The listing builds one solid part. Answer for the finished solid, in the listing's coordinates (mm). A direction names the side the tool comes from. Give positions to 0.01 mm unless a question says otherwise; leave off trailing zeros. Loops run counter-clockwise (first coordinate to the right, second up) from the corner with the lowest first, then second, coordinate; pieces in that order, holes last. Notation, with made-up numbers: M 35.5,-10.5 L 40.5,-10.5 A26 cw 40.5,16.5 Z; hole C 19.5,15.5 d2. An arc over 180 degrees is marked long. One line per item, written item: value. Start each with the question number.
Q1. Consider L1, parallel to Z at x = -1, y = -10; L2, parallel to Z at x = 24, y = 6; L3, parallel to Y at x = 0, z = -9.8. Determine where each line is inside the solid, lowest interval first.
Q2. Flat-ended cylindrical pins translate along their axes: pin 1 (1.5 mm diameter, centred on y = -2, z = -5.5, fed in from -X); pin 2 (2.5 mm diameter, centred on x = 69.5, y = 0.5, fed in from +Z) (3 decimals); pin 3 (6.5 mm diameter, centred on x = 52, z = -4, fed in from +Y). Find the tip coordinate at first contact, or state that the pin passes through.
Q3. A cutting plane is placed at B-B, the plane y = 10.5. Determine the outline of the cut face in (x, z).
Q4. The mould has two halves that part along X. Classify faces 4 (the flat face through (6, 12.5, 2)), 5 (the flat face through (118, -3.2, -2.4)), 6 (the flat face through (48.56, -4.54, 1)): +X half, -X half, draft (parallel to the pull), parting line (faces both ways), or undercut.
Q5. For faces 1 (the flat face through (80, -1.5, 1)), 2 (the flat face through (81, 2, -0.35)), 3 (the flat face through (76, 0, -6.525)), determine the directions among +Z, -Z, +X, -X, +Y, -Y from which every point of the face is accessible in a straight line to the end or side of a thin tool.
Q6. A cutting plane is placed at A-A, the plane x = 96.5. Determine the outline of the cut face in (y, z) (3 decimals).
from build123d import *
from OCP.BRepFilletAPI import BRepFilletAPI_MakeChamfer
from build123d.topology import SkipClean

# Parameters (mm, degrees)
SKETCH1_R           = 7.0625
BOSS_EXTRUDE1_DEPTH = 4
SKETCH5_W           = 25.521905645
SKETCH5_H           = 15
BOSS_EXTRUDE2_DEPTH = 12.7
FILLET1_R           = 7.5
SKETCH6_W           = 64.371907972
SKETCH6_H           = 15
BOSS_EXTRUDE3_DEPTH = 2
CHAMFER1_SIZE       = 10
CHAMFER1_SIZE2      = 6
CHAMFER2_SIZE       = 6
CHAMFER2_SIZE2      = 10
SKETCH8_R           = 2.9375
BOSS_EXTRUDE4_DEPTH = 5
BOSS_EXTRUDE5_DEPTH = 1.5
CUT_EXTRUDE1_DEPTH  = 7.5
SKETCH11_W          = 6.742622272
SKETCH11_H          = 8.688704154
BOSS_EXTRUDE7_DEPTH = 8
FILLET2_R           = 2.5
SKETCH12_R          = 12.5
SKETCH12_R_2        = 7.0625
BOSS_EXTRUDE8_DEPTH = 1.5


# Some blends are built 0.0001 mm under size
with BuildPart() as part:
    # Sketch1 → Boss-Extrude1 (new body)
    with BuildSketch(Plane.XY):
        with BuildLine():
            Line((0, 12.5), (12.041321952, 12.5))
            Line((12.041321952, 12.5), (28.106186383, 7.5))
            Line((28.106186383, 7.5), (28.106186383, -7.5))
            Line((28.106186383, -7.5), (12.041321952, -12.5))
            Line((12.041321952, -12.5), (0, -12.5))
            ThreePointArc((0, -12.5), (-12.5, 0), (0, 12.5))
        make_face()
        Circle(SKETCH1_R, mode=Mode.SUBTRACT)
    boss_extrude1 = extrude(amount=BOSS_EXTRUDE1_DEPTH)

    # Sketch5 → Boss-Extrude2 (add)
    with BuildSketch(Plane.XY.offset(4)):
        with Locations((40.867139206, 0)):
            Rectangle(SKETCH5_W, SKETCH5_H)
    extrude(amount=-BOSS_EXTRUDE2_DEPTH)

    # Mirror1: Boss-Extrude1 across plane
    add(boss_extrude1.mirror(Plane(origin=(0, 0, -2.35), x_dir=(1, 0, 0), z_dir=(0, 0, -1))))

    # Fillet1
    fillet1_edges = [part.edges().sort_by_distance(p)[0] for p in [
        (28.106186383, -7.5, -2.35),
        (28.106186383, 7.5, -2.35),
    ]]
    fillet(fillet1_edges, radius=FILLET1_R - 0.0001)  # a hair under: the kernel refuses the full size

    # Sketch6 → Boss-Extrude3 (add, symmetric)
    with BuildSketch(Plane(origin=(0, 0, -2.35), x_dir=(-1, 0, 0), z_dir=(0, 0, -1))):
        with Locations((-85.814046014, 0)):
            Rectangle(SKETCH6_W, SKETCH6_H)
    extrude(amount=BOSS_EXTRUDE3_DEPTH, both=True)

    # Chamfer1
    chamfer1_edges = [part.edges().sort_by_distance(p)[0] for p in [
        (53.628092028, 7.5, -6.525),
        (53.628092028, 7.5, 1.825),
    ]]
    chamfer1_side = [part.faces().sort_by_distance(p)[0] for p in [
        (62.630754808, 7.5, -2.35),
    ]]
    chamfer(chamfer1_edges, length=CHAMFER1_SIZE, length2=CHAMFER1_SIZE2, reference=chamfer1_side[0])

    # Chamfer2: one chamfer whose edges measure the first distance from different faces: ONE call of the kernel's chamfer builder (chamfer() names one face for all edges)
    chamfer2_edges_1 = [part.edges().sort_by_distance(p)[0] for p in [
        (53.628092028, -7.5, -6.525),
    ]]
    chamfer2_side_1 = [part.faces().sort_by_distance(p)[0] for p in [
        (53.628092028, -3, -6.525),
    ]]
    chamfer2_edges_2 = [part.edges().sort_by_distance(p)[0] for p in [
        (53.628092028, -7.5, 1.825),
    ]]
    chamfer2_side_2 = [part.faces().sort_by_distance(p)[0] for p in [
        (53.628092028, -3, 1.825),
    ]]
    chamfer2 = BRepFilletAPI_MakeChamfer(part.part.solid().wrapped)
    for e in chamfer2_edges_1:
        chamfer2.Add(CHAMFER2_SIZE, CHAMFER2_SIZE2, e.wrapped, chamfer2_side_1[0].wrapped)  # the first distance lies on this face
    for e in chamfer2_edges_2:
        chamfer2.Add(CHAMFER2_SIZE, CHAMFER2_SIZE2, e.wrapped, chamfer2_side_2[0].wrapped)  # the first distance lies on this face
    add(Compound.cast(chamfer2.Shape()), mode=Mode.REPLACE)

    # Sketch8 → Boss-Extrude4 (add)
    with BuildSketch(Plane(origin=(118, 0, 0), x_dir=(0, 0, -1), z_dir=(1, 0, 0))):
        with Locations(Location((2.35, 0, 0), (0, 0, 132.910184022))):
            Circle(SKETCH8_R)
    extrude(amount=BOSS_EXTRUDE4_DEPTH)

    # Sketch9 → Boss-Extrude5 (add, symmetric)
    with BuildSketch(Plane(origin=(0, 0, 0), x_dir=(1, 0, 0), z_dir=(0, 1, 0))):
        Polygon((53.628092028, 6.525), (98.349917778, 6.525), (112.85605343, 2.35), (98.349917778, -1.825), (53.628092028, -1.825), align=None)
    extrude(amount=BOSS_EXTRUDE5_DEPTH, both=True)

    # Sketch10 → Cut-Extrude1 (cut, symmetric)
    with BuildSketch(Plane(origin=(0, 0, 0), x_dir=(1, 0, 0), z_dir=(0, 1, 0))):
        Polygon((53.628092028, 6.525), (35.842858925, 8.7), (53.628092028, 8.7), align=None)
        Polygon((53.628092028, -1.825), (35.842858925, -4), (53.628092028, -4), align=None)
    extrude(amount=CUT_EXTRUDE1_DEPTH, both=True, mode=Mode.SUBTRACT)

    # Sketch11 → Boss-Extrude7 (add)
    with BuildSketch(Plane.ZY.offset(-118)):
        with Locations((-2.35, 0)):
            Rectangle(SKETCH11_W, SKETCH11_H)
    extrude(amount=BOSS_EXTRUDE7_DEPTH)

    # Fillet2
    # the kernel refuses this fillet: 2.5 mm, written as the material it takes off along each edge
    with BuildSketch(Plane(origin=(123.576771831, 4.344352077, 1.021311136), x_dir=(0, -1, 0), z_dir=(-1, 0, 0)), Plane(origin=(123.576771831, -4.344352077, -5.721311136), x_dir=(0, 1, 0), z_dir=(-1, 0, 0))) as fillet2_piece_1:
        with BuildLine():
            CenterArc((2.230708732, -2.5), FILLET2_R, 90, 63.161607103)
            Line((0, -1.371311136), (-0.044614175, -1.348737359))
            ThreePointArc((-0.044614175, -1.348737359), (-0.05, -0.685655568), (-0.05, 0))
            Line((-0.05, 0), (0, 0.05))
            Line((0, 0.05), (2.230708732, 0.05))
            Line((2.230708732, 0.05), (2.230708732, 0))
        make_face()
    extrude(amount=19.153543662, mode=Mode.SUBTRACT)
    with BuildSketch(Plane(origin=(123.576771831, -4.344352077, 1.021311136), x_dir=(0, 0, -1), z_dir=(-1, 0, 0)), Plane(origin=(123.576771831, 4.344352077, -5.721311136), x_dir=(0, 0, 1), z_dir=(-1, 0, 0))) as fillet2_piece_2:
        with BuildLine():
            CenterArc((2.5, -2.230708732), FILLET2_R, 116.838392897, 63.161607103)
            Line((0, -2.230708732), (-0.05, -2.230708732))
            Line((-0.05, -2.230708732), (-0.05, 0))
            Line((-0.05, 0), (0, 0.05))
            ThreePointArc((0, 0.05), (0.685655568, 0.05), (1.348737359, 0.044614175))
            Line((1.348737359, 0.044614175), (1.371311136, 0))
        make_face()
    extrude(amount=19.153543662, mode=Mode.SUBTRACT)

    # Sketch12 → Boss-Extrude8 (add)
    with SkipClean():  # the faces are left unmerged after this step: merging them gives an invalid solid
        with BuildSketch(Plane(origin=(0, 0, -8.7), x_dir=(-1, 0, 0), z_dir=(0, 0, -1))):
            with Locations(Location((0, 0, 0), (0, 0, 90))):
                Circle(SKETCH12_R)
            with Locations(Location((0, 0, 0), (0, 0, 180))):
                Circle(SKETCH12_R_2, mode=Mode.SUBTRACT)
        boss_extrude8 = extrude(amount=BOSS_EXTRUDE8_DEPTH)

    # Mirror2: Boss-Extrude8 across plane
    with SkipClean():  # the faces are left unmerged after this step: merging them gives an invalid solid
        add(boss_extrude8.mirror(Plane(origin=(0, 0, -2.35), x_dir=(1, 0, 0), z_dir=(0, 0, -1))))


solid = part.part
Answer block:
1. L1: -10.2 to -4.7, 0 to 5.5
1. L2: -8.7 to -4.7, 0 to 4
1. L3: -12.5 to -7.06, 7.06 to 12.5
2. pin 1: x = -12.44
2. pin 2: z = 1.825
2. pin 3: y = 7.5
3. outline: M -6.78,-10.2 L 6.78,-10.2 L 6.78,-8.7 L 18.47,-8.7 L 18.47,-4.7 L -6.78,-4.7 Z; M -6.78,0 L 18.47,0 L 18.47,4 L 6.78,4 L 6.78,5.5 L -6.78,5.5 Z
4. face 4: draft
4. face 5: +X half
4. face 6: undercut
5. face 1: +Z, -Y
5. face 2: +Z
5. face 3: -Z, +X, +Y, -Y
6. outline: M -7.5,-4.35 L -1.5,-4.35 L -1.5,-6.525 L 1.5,-6.525 L 1.5,-4.35 L 7.5,-4.35 L 7.5,-0.35 L 1.5,-0.35 L 1.5,1.825 L -1.5,1.825 L -1.5,-0.35 L -7.5,-0.35 Z
